```python
from build123d import *

# Parameters (mm, degrees)
F0_W           = 61.9914149866
F0_H           = 40.331762284
F1_DEPTH       = 20.32
F2_DEPTH       = 15.24
F5_R           = 4.1121060328
F6_DEPTH       = 20.32
F7_W           = 14.0040833503
F7_H           = 6.9086803123
F8_DEPTH       = 17.78
F9_W           = 15.3111321852
F9_H           = 14.2841655761
F10_DEPTH      = 61.9924149866
F10_DEPTH_BACK = 25.4
F11_W          = 10.2332767595
F11_H          = 6.8242249937
F12_DEPTH      = 35.561
F13_W          = 34.0766059235
F13_H          = 30.1554612815
F14_DEPTH      = 35.561


# Not quite as in the source:
# - the program builds the solid bodies; features that only make, move or delete a surface that nothing else refers to are left out


with BuildPart() as f1:
    # F0 (on Front) → F1 (new body)
    with BuildSketch(Plane.XZ):
        with Locations((-3.0808984302, 9.9895801395)):
            Rectangle(F0_W, F0_H)
    extrude(amount=F1_DEPTH)

    # F2 (add): a face of the model
    f2_faces = [f1.faces().sort_by_distance(p)[0] for p in [
        (-3.0808984302, -20.32, 9.9895801395),
    ]]
    extrude(f2_faces, amount=F2_DEPTH)

    # F5 (on face) → F6 (cut)
    with BuildSketch(Plane.XZ.offset(35.56)):
        Circle(F5_R)
    extrude(amount=-F6_DEPTH, mode=Mode.SUBTRACT)

    # F7 (on face) → F8 (cut)
    with BuildSketch(Plane.XY.offset(30.1554612815)):
        with Locations((-4.4813072309, -16.991621349)):
            Rectangle(F7_W, F7_H)
    extrude(amount=-F8_DEPTH, mode=Mode.SUBTRACT)

    # F9 (on face) → F10 (cut, two sides)
    with BuildSketch(Plane.YZ.offset(27.9148090631)) as f10_sk:
        with Locations((-15.7779348083, 7.1420827881)):
            Rectangle(F9_W, F9_H)
    extrude(amount=-F10_DEPTH, mode=Mode.SUBTRACT)
    extrude(f10_sk.sketch, amount=F10_DEPTH_BACK, mode=Mode.SUBTRACT)

    # F11 (on face) → F12 (cut, through all)
    with BuildSketch(Plane.XZ.offset(35.56)):
        with Locations((22.7981706833, 26.7433487847)):
            Rectangle(F11_W, F11_H)
    extrude(amount=-F12_DEPTH, mode=Mode.SUBTRACT)

    # F13 (on face) → F14 (cut, through all)
    with BuildSketch(Plane.XZ):
        with Locations((-17.0383029617, 15.0777306408)):
            Rectangle(F13_W, F13_H)
    extrude(amount=F14_DEPTH, mode=Mode.SUBTRACT)


solid = f1.part
```
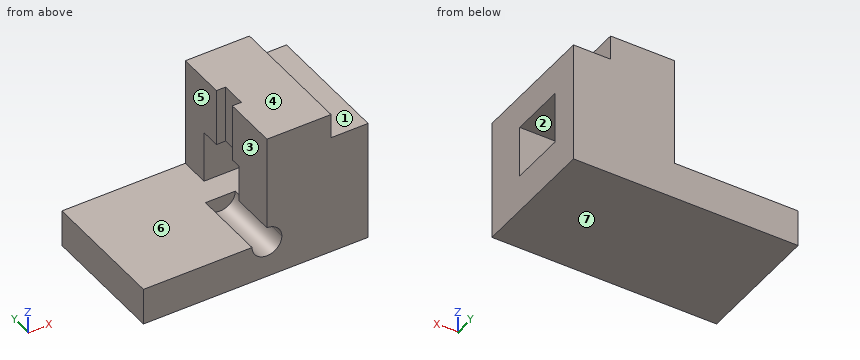
Read the model definition and answer for the solid it produces. Units are mm, in the model's axes. Face numbers are marked on the shaded views. A direction names the side the tool comes from. Coordinates: 2 decimals unless noted, no trailing zeros. Loops run counter-clockwise (first coordinate to the right, second up) from the corner with the lowest first, then second, coordinate; pieces in that order, holes last.
(1) Consider line 1 along Z through (x, y) = (16.5, -8.5); line 2 along Y through (x, z) = (16, 10.5); line 3 along X through (y, z) = (-27, 11.5). Determine where each line is inside the solid, lowest interval first.
Solution:
line 1: z = -10.18 to 0, 14.28 to 30.16
line 2: y = -35.56 to -23.43, -8.12 to 0
line 3: x = 0 to 27.91
(2) The part is cut by section D-D (y = -29). Determine the outline of the cut face in (x, z).
Solution:
outline: (-34.08, -10.18) - (27.91, -10.18) - (27.91, 23.33) - (17.68, 23.33) - (17.68, 30.16) - (0, 30.16) - (0, 4.11) arc R4.11 cw (long way) to (-4.11, 0) - (-34.08, 0) - close
(3) The part is cut by section A-A (z = 12). Determine the outline of the cut face in (x, y).
Solution:
outline: (0, -35.56) - (27.91, -35.56) - (27.91, -23.43) - (0, -23.43) - close; (0, -8.12) - (27.91, -8.12) - (27.91, 0) - (0, 0) - close
(4) A tool of negligible diameter and unlimited length cuts with its end or side. For the marked faces 1, 2, 3 and 4, from which of +Z, -Z, +X, -X, +Y, -Y can it reach the whole face along a straight path? Write none if from no direction.
Solution:
face 1: +Z, +X, +Y, -Y
face 2: +X, -X
face 3: +Z, -X, +Y, -Y
face 4: +Z, +X, -X, +Y, -Y
(5) The mould has two halves that part along Z. Classify the marked faces 5, 6 and 7: released by +Z, released by -Z, zero draft, split by the parting line, or undercut.
Solution:
face 5: zero draft
face 6: undercut
face 7: released by -Z
(6) The part is cut by section C-C (x = 13). Determine the outline of the cut face in (y, z).
Solution:
outline: (-35.56, -10.18) - (0, -10.18) - (0, 30.16) - (-35.56, 30.16) - close; hole (-23.43, 0) - (-8.12, 0) - (-8.12, 14.28) - (-23.43, 14.28) - close
(7) Flat-ended cylindrical pins translate along their axes: pin 1 Ø2 at (y, z) = (-19.5, 25.5) entering from -X; pin 2 Ø2 at (y, z) = (-20.5, 25.5) entering from +X; pin 3 Ø12 at (x, y) = (-19.5, -22.5) entering from +Z. Find the tip coordinate at first contact, or state that the pin passes through.
Solution:
pin 1: stops at x = 0
pin 2: stops at x = 17.68
pin 3: stops at z = 0
(8) The part is cut by section B-B (y = -9). Determine the outline of the cut face in (x, z).
Solution:
outline: (-34.08, -10.18) - (27.91, -10.18) - (27.91, 0) - (-34.08, 0) - close; (0, 14.28) - (27.91, 14.28) - (27.91, 23.33) - (17.68, 23.33) - (17.68, 30.16) - (0, 30.16) - close
